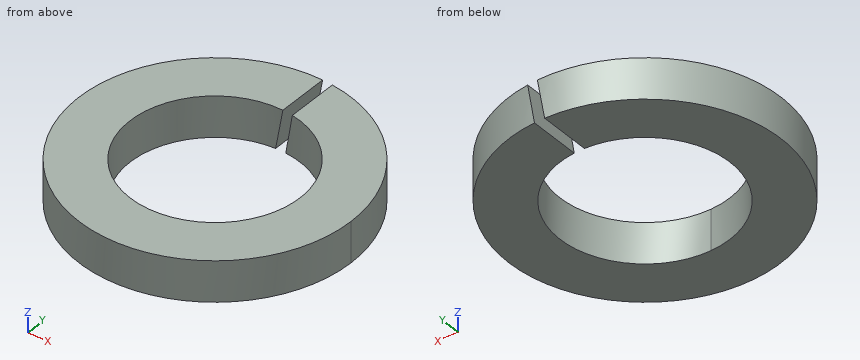
Autodesk Inventor part; units mm, degrees
ref_plane "WorkPlane1" through (0, 0, 0) normal (0, 0, 1) x (1, 0, 0)
ref_plane "WorkPlane3" through (0, 0, -5.94) normal (0, 0, 1) x (1, 0, 0)
ref_plane "Work Plane3" through (0, -19.895, 0) normal (0, 1, 0) x (-1, 0, 0)
ref_plane "WorkPlane1" through (0, 0, 0) normal (0, 0, 1) x (1, 0, 0)
ref_plane "WorkPlane3" through (0, 0, -5.94) normal (0, 0, 1) x (1, 0, 0)
ref_plane "Work Plane3" through (0, -19.895, 0) normal (0, 1, 0) x (-1, 0, 0)
ref_plane "WorkPlane10" through (0, 19.895, 0) normal (0, 1, 0) x (-1, 0, 0)
sketch "Sketch1" plane through (0, 0, 0) normal (0, 0, 1) x (1, 0, 0)
  point P0 (0, 0)
sketch "Sketch2" plane through (0, 0, 0) normal (0, 0, 1) x (1, 0, 0)
  circle A0 centre (0, 0) radius 19.895
  dimension "d3" = 39.79
extrude "Extrusion1" add sketch "Sketch2" against normal blind 5.94
sketch "Sketch3" plane through (0, 0, -5.94) normal (0, 0, 1) x (1, 0, 0)
  point P0 (0, 0)
sketch "Sketch4" plane through (0, 0, 0) normal (0, 0, 1) x (1, 0, 0)
  circle A0 centre (0, 0) radius 19.895
hole "Hole1" at (0, 0, 0) direction (0, 0, -1) diameter 24.81 end through all
sketch "Sketch5" plane through (0, 19.895, 0) normal (0, 1, 0) x (-1, 0, 0)
  line L0 (-0.3049, 0) -> (-1.7899, 0)
  line L1 (0.7425, -5.94) -> (-0.3049, 0)
  line L2 (-0.7425, -5.94) -> (0.7425, -5.94)
  line L3 (-1.7899, 0) -> (-0.7425, -5.94)
  line L4 (-12.405, 0) -> (12.405, 0) construction
  line L5 (19.895, -5.94) -> (-19.895, -5.94) construction
  line L6 (0, -7.128) -> (0, 1.188)
  dimension "d15" = 80
  dimension "d18" = 0.7425
  dimension "d19" = 0.7425
extrude "Extrusion2" cut sketch "Sketch5" against normal blind 19.895
ref_plane "MSC_PT1" through (0, 0, 0) normal (0, 0, 1) x (1, 0, 0)
ref_plane "MSC_PT2" through (0, 0, -5.94) normal (0, 0, -1) x (-1, 0, 0)
equation "\"d7\" = Diam1"
equation "\"d4\" = ParH"
equation "\"d18\" = 0.125 * ParH"
equation "\"d19\" = 0.125 * ParH"
equation "\"d16\" = 0.5 * Diam2"
equation "\"d3\" = Diam2"
equation "\"Diam2\" = 39.79"
equation "\"ParH\" = 5.94"
equation "\"Diam1\" = 24.81"
equation "\"d20\" = 0.5 * Diam2"
properties part number "ASME B18.21.2M - 24" material "Steel, Mild"
CAD build for the part. Positions are in the model's coordinates, mm. Coordinates: 2 decimals unless noted, no trailing zeros. Order: outer loops, then holes, each group sorted by start corner. A loop starts at its lowest first (then second) coordinate and runs counter-clockwise, first axis right, second up. Notation, with made-up numbers: (5, 70) - (25, 70) arc R21 ccw to (25, 92) - close; hole circle Ø10 at (61.25, 10.25). An arc over 180 degrees is marked (long way). Use a Markdown table: item, result. Add a question column.
(1) Flat gauge pins, fed straight in: pin 1 (1 mm diameter, centred on y = 9.5, z = -1.5, fed in from +X); pin 2 (3 mm diameter, centred on x = 5.5, y = -8.5, fed in from +Z); pin 3 (1.5 mm diameter, centred on y = -4, z = -0.5, fed in from -X); pin 4 (1 mm diameter, centred on x = 3, z = -3.5, fed in from -Y). Where does each tip first touch, or does it go through?
(2) Saw through at C-C (z = -3.2). Give the cut face in (x, y) (3 decimals).
(3) Saw through at B-B (y = -1.5). Give the cut face in (x, z), then the cut area to 3 significant figures.
(4) Saw through at A-A (x = 9). Give the cut face in (y, z).
(5) Saw through at D-D (x = 14.5). Give the cut face in (y, z), then the cut area to 3 significant figures.
(6) Drill centre lines: line 1 along Y through (x, z) = (-10, -0.5); line 2 along X through (y, z) = (9.5, -2.5); line 3 along Y through (x, z) = (0, -4.2) (3 decimals). Where is each one in solid material? Low to high. Write a range as [from, to].
Solved:
| question | item | result |
|---|---|---|
| 1 | pin 1 | stops at x = 17.74 |
| 1 | pin 2 | passes through |
| 1 | pin 3 | stops at x = -19.63 |
| 1 | pin 4 | stops at y = -19.74 |
| 2 | outline | (-0.259, 12.402) - (-0.259, 19.893) arc R19.895 ccw (long way) to (1.226, 19.857) - (1.226, 12.344) arc R12.405 cw (long way) to start |
| 3 | outline | (-19.84, -5.94) - (-12.31, -5.94) - (-12.31, 0) - (-19.84, 0) - close; (12.31, -5.94) - (19.84, -5.94) - (19.84, 0) - (12.31, 0) - close |
| 3 | area | 89.4 mm² |
| 4 | outline | (-17.74, -5.94) - (-8.54, -5.94) - (-8.54, 0) - (-17.74, 0) - close; (8.54, -5.94) - (17.74, -5.94) - (17.74, 0) - (8.54, 0) - close |
| 5 | outline | (-13.62, -5.94) - (13.62, -5.94) - (13.62, 0) - (-13.62, 0) - close |
| 5 | area | 162 mm² |
| 6 | line 1 | y = [-17.2, -7.34], [7.34, 17.2] |
| 6 | line 2 | x = [-17.48, -7.98], [7.98, 17.48] |
| 6 | line 3 | y = [-19.895, -12.405] |
